```python
from build123d import *

# Parameters (mm, degrees)
EXTRUDE_1_DEPTH = 10


with BuildPart() as part:
    # ｽｹｯﾁ1 → ﾎﾞｽ - 押し出し1 (new body)
    with BuildSketch(Plane.XY):
        with BuildLine():
            Line((4, -3.1), (4, 3.1))
            Line((4, 3.1), (6, 3.1))
            Line((6, 3.1), (6, 5.1))
            Line((6, 5.1), (0.8, 5.1))
            Line((0.8, 5.1), (0.8, 3))
            Line((0.8, 3), (0.8, 2.631064423))
            ThreePointArc((0.8, 2.631064423), (2.75, 0), (0.8, -2.631064423))
            Line((0.8, -2.631064423), (0.8, -3))
            Line((0.8, -3), (0.8, -5.1))
            Line((0.8, -5.1), (6, -5.1))
            Line((6, -5.1), (6, -3.1))
            Line((6, -3.1), (4, -3.1))
        make_face()
    extrude(amount=EXTRUDE_1_DEPTH)


solid = part.part
```
Model file for the job. Use its own axes, mm. A direction names the side the tool comes from. Coordinates: 2 decimals unless noted, no trailing zeros. Loops run counter-clockwise (first coordinate to the right, second up) from the corner with the lowest first, then second, coordinate; pieces in that order, holes last. Notation, with made-up numbers: (24, 74) - (32, 74) arc R27 cw to (32, 113) - close; hole circle Ø11 at (-38, 15.25). An arc over 180 degrees is marked (long way). Write item = value, one per line. Start each with the question number.
Item 1: Saw through at D-D, the plane y = 1.25. List the corners of the cut face in (x, z), then the cut area to 3 significant figures.
Item 2: Saw through at B-B, the plane z = 6. List the corners of the cut face in (x, y).
Item 3: Saw through at C-C, the plane x = 1.8. List the corners of the cut face in (y, z), then the cut area to 3 significant figures.
Item 4: Saw through at A-A, the plane x = 4.7. List the corners of the cut face in (y, z), then the cut area to 3 significant figures.
Item 5: 3-axis set-ups, long thin cutter, end or side, ignore diameter. For faces 1 (the face through (4, 0, 5)), 2 (the face through (0.8, -4, 5)): which of +Z, -Z, +X, -X, +Y, -Y reach the whole face in a straight line?
Item 6: Wall check: probe 1 along Y at (x, z) = (5.5, 5.5); probe 2 along Y at (x, z) = (1.9, 4.25); probe 3 along X at (y, z) = (-1.5, 7.5). Give the ranges that are in metal, low to high. Write a range as [from, to].
Item 7: Drop a flat-ended pin along its axis: pin 1 Ø1 at (y, z) = (1, 6.5) entering from -X. Give the stop position or say it passes through.
Answers:
q1.outline = (2.45, 0) - (4, 0) - (4, 10) - (2.45, 10) - close
q1.area = 15.5 mm2
q2.outline = (0.8, -5.1) - (6, -5.1) - (6, -3.1) - (4, -3.1) - (4, 3.1) - (6, 3.1) - (6, 5.1) - (0.8, 5.1) - (0.8, 2.63) arc R2.75 cw to (0.8, -2.63) - close
q3.outline = (-5.1, 0) - (-2.08, 0) - (-2.08, 10) - (-5.1, 10) - close; (2.08, 0) - (5.1, 0) - (5.1, 10) - (2.08, 10) - close
q3.area = 60.4 mm2
q4.outline = (-5.1, 0) - (-3.1, 0) - (-3.1, 10) - (-5.1, 10) - close; (3.1, 0) - (5.1, 0) - (5.1, 10) - (3.1, 10) - close
q4.area = 40.0 mm2
q5.face_1 = +Z, -Z, +X
q5.face_2 = +Z, -Z, -X, +Y, -Y
q6.probe_1 = [-5.1, -3.1], [3.1, 5.1]
q6.probe_2 = [-5.1, -1.99], [1.99, 5.1]
q6.probe_3 = [2.3, 4]
q7.pin_1 = 2.3
